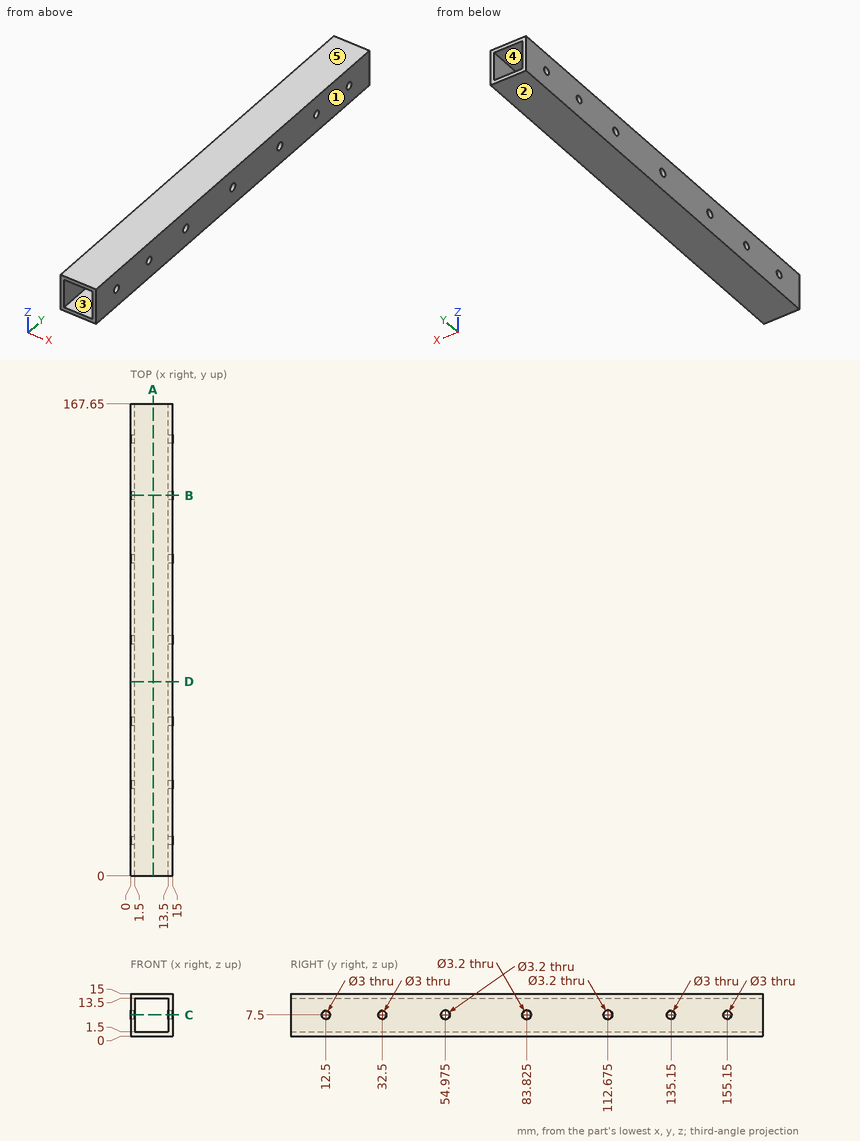
The drawing under review shows one solid part. Ordinate dimensions are in mm from its lowest x, y, z. A direction names the side the tool comes from. Round coordinates to 2 decimals unless told otherwise and drop trailing zeros. Loops run counter-clockwise (first coordinate to the right, second up) from the corner with the lowest first, then second, coordinate; pieces in that order, holes last. Notation, with made-up numbers: (35, 39) -> (65, 39) arc R21 cw to (65, 64) -> close; hole circle Ø7 at (56.25, -3). An arc over 180 degrees is marked (long way). One line per question, with ' | ' between items. Start each with the question number.
Item 1: Machinability: for the marked faces 4 and 5, which of the approach directions +Z, -Z, +X, -X, +Y, -Y give a long, thin tool a straight path to every point of the face, cutting with its end or side? Answer none if there is none.
Item 2: Add section A-A, the plane x = 8. Write out the cut boundary in (y, z).
Item 3: Wall thickness on line 1 along Z through (x, y) = (10.75, 22.5); line 2 along Z through (x, y) = (14.65, 135.15): over which ranges is each line inside the solid? List them lowest first. Write a range as [from, to].
Item 4: Add section B-B, the plane y = 135.15. Write out the cut boundary in (x, z).
Item 5: Draft analysis for pull direction X (two halves, no side actions). For the marked faces 1, 2 and 3, state which applies: +X half, -X half, draft (parallel to the pull), parting line (faces both ways), or undercut.
Item 6: For pin 1 (2 mm diameter, centred on x = 12, z = 11.5, fed in from -Y), flat-tipped, find the tip position at first contact; note if it passes through.
Item 7: Add section D-D, the plane y = 69. Write out the cut boundary in (x, z), then the cut area to 3 significant figures.
Item 8: Add section C-C, the plane z = 7.5. Count the separate pieces of the cut face and the enclosed holes in it, then the cut area to 3 significant figures.
Return value:
1) face 4: +Y, -Y | face 5: +Z, +X, -X, +Y, -Y
2) outline: (0, 0) -> (167.65, 0) -> (167.65, 1.5) -> (0, 1.5) -> close; (0, 13.5) -> (167.65, 13.5) -> (167.65, 15) -> (0, 15) -> close
3) line 1: z = [0, 1.5], [13.5, 15] | line 2: z = [0, 6], [9, 15]
4) outline: (0, 0) -> (15, 0) -> (15, 6) -> (13.5, 6) -> (13.5, 1.5) -> (1.5, 1.5) -> (1.5, 6) -> (0, 6) -> close; (0, 9) -> (1.5, 9) -> (1.5, 13.5) -> (13.5, 13.5) -> (13.5, 9) -> (15, 9) -> (15, 15) -> (0, 15) -> close
5) face 1: +X half | face 2: draft | face 3: undercut
6) pin 1: passes through
7) outline: (0, 0) -> (15, 0) -> (15, 15) -> (0, 15) -> close; hole (1.5, 1.5) -> (13.5, 1.5) -> (13.5, 13.5) -> (1.5, 13.5) -> close | area: 81.0 mm2
8) separate pieces: 16 | enclosed holes: 0 | area: 438 mm2
